from build123d import *

# Parameters (mm, degrees)
BOSS_EXTRUDE1_DEPTH = 227.56368
SKETCH9_R           = 6.35
CUT_EXTRUDE2_DEPTH  = 3.048


with BuildPart() as part:
    # Sketch4 → Boss-Extrude1 (new body)
    with BuildSketch(Plane.XY):
        with BuildLine():
            Line((25.4, -16.51), (25.4, 16.51))
            ThreePointArc((25.4, 16.51), (24.656051224, 18.306051224), (22.86, 19.05))
            Line((22.86, 19.05), (-22.86, 19.05))
            ThreePointArc((-22.86, 19.05), (-24.656051224, 18.306051224), (-25.4, 16.51))
            Line((-25.4, 16.51), (-25.4, -16.51))
            ThreePointArc((-25.4, -16.51), (-24.656051224, -18.306051224), (-22.86, -19.05))
            Line((-22.86, -19.05), (22.86, -19.05))
            ThreePointArc((22.86, -19.05), (24.656051224, -18.306051224), (25.4, -16.51))
        make_face()
        with BuildLine():
            Line((22.352, 14.4018), (22.352, -14.4018))
            ThreePointArc((22.352, -14.4018), (21.883312271, -15.533312271), (20.7518, -16.002))
            Line((20.7518, -16.002), (-20.7518, -16.002))
            ThreePointArc((-20.7518, -16.002), (-21.883312271, -15.533312271), (-22.352, -14.4018))
            Line((-22.352, -14.4018), (-22.352, 14.4018))
            ThreePointArc((-22.352, 14.4018), (-21.883312271, 15.533312271), (-20.7518, 16.002))
            Line((-20.7518, 16.002), (20.7518, 16.002))
            ThreePointArc((20.7518, 16.002), (21.883312271, 15.533312271), (22.352, 14.4018))
        make_face(mode=Mode.SUBTRACT)
    extrude(amount=BOSS_EXTRUDE1_DEPTH)

    # Sketch9 → Cut-Extrude2 (cut)
    with BuildSketch(Plane(origin=(0, 19.05, 0), x_dir=(1, 0, 0), z_dir=(0, 1, 0))):
        with Locations((0, -139.18184)):
            Circle(SKETCH9_R)
        with Locations((0, -88.38184)):
            Circle(SKETCH9_R)
    extrude(amount=-CUT_EXTRUDE2_DEPTH, mode=Mode.SUBTRACT)


solid = part.part
The model under review builds one solid part; all positions refer to its coordinate system, in mm. A direction names the side the tool comes from. Coordinates: 2 decimals unless noted, no trailing zeros. Order: outer loops, then holes, each group sorted by start corner. A loop starts at its lowest first (then second) coordinate and runs counter-clockwise, first axis right, second up. Notation, with made-up numbers: (62, 40) -> (95, 40) arc R23 cw to (95, 48) -> close; hole circle Ø5 at (44.5, -12.75). An arc over 180 degrees is marked (long way). Answer in a Markdown table with one row per item.
(1) Wall thickness on line 1 along Z through (x, y) = (0, 17.15); line 2 along X through (y, z) = (-11, 121); line 3 along Y through (x, z) = (-6.5, 152.5): over which ranges is each line inside the solid? List them lowest first.
Answers:
| item | result |
|---|---|
| line 1 | 0 to 82.03, 94.73 to 132.83, 145.53 to 227.56 |
| line 2 | -25.4 to -22.35, 22.35 to 25.4 |
| line 3 | -19.05 to -16, 16 to 19.05 |
(2) Consider section B-B (y = -12.5). Write out the cut boundary in (x, z), plus the area to 3 significant figures.
Answers:
| item | result |
|---|---|
| outline | (-25.4, 0) -> (-22.35, 0) -> (-22.35, 227.56) -> (-25.4, 227.56) -> close; (22.35, 0) -> (25.4, 0) -> (25.4, 227.56) -> (22.35, 227.56) -> close |
| area | 1,390 mm² |
(3) The part is to be moulded in two halves that separate along X. For faces 1 (the flat face through (25.4, 0, 112)), 2 (the flat face through (0, 16.002, 112)), 3 (the flat face through (2, -17, 0)), 4 (the flat face through (0, -16.002, 112)), say which applies: +X half, -X half, draft (parallel to the pull), parting line (faces both ways), or undercut.
Answers:
| item | result |
|---|---|
| face 1 | +X half |
| face 2 | undercut |
| face 3 | draft |
| face 4 | undercut |
(4) Consider section A-A (x = 0). Write out the cut boundary in (y, z).
Answers:
| item | result |
|---|---|
| outline | (-19.05, 0) -> (-16, 0) -> (-16, 227.56) -> (-19.05, 227.56) -> close; (16, 0) -> (19.05, 0) -> (19.05, 82.03) -> (16, 82.03) -> close; (16, 94.73) -> (19.05, 94.73) -> (19.05, 132.83) -> (16, 132.83) -> close; (16, 145.53) -> (19.05, 145.53) -> (19.05, 227.56) -> (16, 227.56) -> close |
(5) Consider section D-D (z = 161). Write out the cut boundary in (x, y).
Answers:
| item | result |
|---|---|
| outline | (-25.4, -16.51) arc R2.54 ccw to (-22.86, -19.05) -> (22.86, -19.05) arc R2.54 ccw to (25.4, -16.51) -> (25.4, 16.51) arc R2.54 ccw to (22.86, 19.05) -> (-22.86, 19.05) arc R2.54 ccw to (-25.4, 16.51) -> close; hole (-22.35, -14.4) arc R1.6 ccw to (-20.75, -16) -> (20.75, -16) arc R1.6 ccw to (22.35, -14.4) -> (22.35, 14.4) arc R1.6 ccw to (20.75, 16) -> (-20.75, 16) arc R1.6 ccw to (-22.35, 14.4) -> close |
(6) Insertion check: pin 1 (6 mm diameter, centred on x = 6, y = -11.5, fed in from +Z). The pin has a flat end and moves straight along its axis. Give the tip position at first contact, or say it passes through.
Answers:
| item | result |
|---|---|
| pin 1 | through |
(7) Consider section C-C (x = -14). Write out the cut boundary in (y, z).
Answers:
| item | result |
|---|---|
| outline | (-19.05, 0) -> (-16, 0) -> (-16, 227.56) -> (-19.05, 227.56) -> close; (16, 0) -> (19.05, 0) -> (19.05, 227.56) -> (16, 227.56) -> close |
(8) Machinability: for faces 5 (the cylindrical face through (-1.38, 17.55, 94.58)), 6 (the flat face through (-22.352, 0, 112)), 7 (the flat face through (0, -19.05, 112)), which of the approach directions +Z, -Z, +X, -X, +Y, -Y give a long, thin tool a straight path to every point of the face, cutting with its end or side? Answer none if there is none.
Answers:
| item | result |
|---|---|
| face 5 | +Y |
| face 6 | +Z, -Z |
| face 7 | +Z, -Z, +X, -X, -Y |
